from build123d import *

# Parameters (mm, degrees)
F0_W     = 80
F0_H     = 70
F1_DEPTH = 60
F2_SIZE  = 20
F4_D     = 15
F6_D     = 15
F6_DEPTH = 15
F6_TIP   = 4.5064546427
F7_R     = 3


with BuildPart() as f1:
    # F0 (on Top) → F1 (new body)
    with BuildSketch(Plane.XY):
        with Locations((-40, -35)):
            Rectangle(F0_W, F0_H)
    extrude(amount=F1_DEPTH)

    # F2
    f2_edges = [f1.edges().sort_by_distance(p)[0] for p in [
        (-40, -70, 60),
    ]]
    chamfer(f2_edges, length=F2_SIZE)

    # F4 (through all)
    with Locations(Plane(origin=(0, -55, 55), x_dir=(1, 0, 0), z_dir=(0, -0.7071067812, 0.7071067812))):
        with Locations((-24, -6.2132034356)):
            Hole(F4_D / 2)

    # F6
    with Locations(Plane(origin=(0, -55, 55), x_dir=(1, 0, 0), z_dir=(0, -0.7071067812, 0.7071067812))):
        with Locations((-59.0175294898, -6.2132034356)):
            Hole(F6_D / 2, depth=F6_DEPTH)
            with Locations((0, 0, -(F6_DEPTH + F6_TIP / 2))):  # 118° drill point
                Cone(0, F6_D / 2, F6_TIP, mode=Mode.SUBTRACT)

    # F7
    f7_edges = [f1.edges().sort_by_distance(p)[0] for p in [
        (0, -35, 0),
    ]]
    fillet(f7_edges, radius=F7_R)


solid = f1.part
Could you check a few things on this model? Use its own coordinates, in mm. A direction names the side the tool comes from. Round coordinates to 2 decimals unless told otherwise and drop trailing zeros. Order: outer loops, then holes, each group sorted by start corner. A loop starts at its lowest first (then second) coordinate and runs counter-clockwise, first axis right, second up. Notation, with made-up numbers: M -2.5,55 L 52.5,55 A15 cw 52.5,64 Z; hole C 87,-18 d7. An arc over 180 degrees is marked long. One line per item, written item: value.
(1) If we mould it in two halves opening along Z, with no side actions, what happens to faces 3 (the flat face through (-41, -60, 50)), 4 (the flat face through (-42, -35, 0)), 5 (the cylindrical face through (-51.525, -53.783, 45.462)), 6 (the flat face through (-41, -70, 20))? For each: released by +Z, released by -Z, zero draft, split by the parting line, or undercut.
Ans:
face 3: released by +Z
face 4: released by -Z
face 5: undercut
face 6: zero draft
(2) Imagine slicing it at A-A (x = -15). Write out the boundary of the cut face in (y, z).
Ans:
outline: M -70,0 L 0,0 L 0,60 L -50,60 L -70,40 Z
(3) Which directions (+Z, -Z, +X, -X, +Y, -Y) give clear straight access to the entire face, cutting with the end or side of a thin tool? Please do faces 1 (the conical face through (-57.814, -46.506, 37.014)), 2 (the flat face through (-41, -25, 60)).
Ans:
face 1: none
face 2: +Z, +X, -X, +Y, -Y
(4) I need wall thicknesses on line 1 along Y through (x, z) = (-19, 36); line 2 along Z through (x, y) = (-26, -37); line 3 along Z through (x, y) = (-59, -52). Which ranges of each line are inside material? Lowest first, please. Write a range as from..to.
Ans:
line 1: y = -70..-52.69, -36.88..0
line 2: z = 0..17.99, 38.44..60
line 3: z = 0..35.22, 53.82..58
(5) I'm going to push flat-ended pins straight in: P1, Ø8, axis at x = -47.5, y = -8.5, coming from the -Z side; P2, Ø3, axis at x = -43.5, y = -52, coming from the +Z side. Where does each tip first touch, or does it pass through?
Ans:
P1: stops at z = 0
P2: stops at z = 59.5
(6) Imagine slicing it at B-B (z = 44). Count the separate pieces of the cut face and the enclosed holes in it, and give its area (3 significant figures).
Ans:
separate pieces: 1
enclosed holes: 2
area: 4,790 mm^2
